Geometry check sheet. Reference: the model listing, model coordinates, mm. Face numbers are marked on the shaded views. A direction names the side the tool comes from. Round coordinates to 2 decimals unless told otherwise and drop trailing zeros. Loops run counter-clockwise (first coordinate to the right, second up) from the corner with the lowest first, then second, coordinate; pieces in that order, holes last.
Autodesk Fusion 360 part; units mm, degrees
sketch "Sketch1" plane through (0, 0, 0) normal (0, 1, 0) x (1, 0, 0)
  line L0 (0, 64.0421) -> (0, -79.964)
  line L1 (-3.05, -8) -> (-3.05, 0)
  line L2 (-6.25, 0) -> (-6.25, 12)
  line L3 (-6.25, 0) -> (-3.05, 0)
  line L4 (-8.05, -8) -> (-8.05, -5)
  line L5 (-11.25, -5) -> (-8.05, -5)
  line L6 (-11.25, -5) -> (-11.25, 12)
  line L7 (-8.05, -8) -> (-3.05, -8)
  line L8 (-11.25, 12) -> (-6.25, 12)
  line L9 (-3.05, -8) -> (0, -7.961)
  line L10 (-6.25, 12) -> (0, 12)
  dimension "d1" = 12.5
  dimension "d2" = 6.1
  dimension "d3" = 8
  dimension "d7" = 12
  dimension "d8" = -5
revolve "Revolve1" add sketch "Sketch1" angle 360 about axis through (0, 0, -64.0421) along (0, 0, 1)
sketch "Sketch2" plane through (0, 0, 8) normal (0, 0, 1) x (-1, 0, 0)
  circle A0 centre (0, 0) radius 3.05 construction
  circle A1 centre (0, 0) radius 8.05
  line L0 (-3.05, 3.05) -> (3.05, 3.05)
  line L1 (3.05, 3.05) -> (3.05, -3.05)
  line L2 (3.05, -3.05) -> (-3.05, -3.05)
  line L3 (-3.05, -3.05) -> (-3.05, 3.05)
  line L4 (-3.05, 3.05) -> (3.05, -3.05) construction
  line L5 (3.05, 3.05) -> (-3.05, -3.05) construction
  point P0 (3.05, 0)
extrude "Extrude1" cut sketch "Sketch2" against normal through all contours L0 L1 L2 L3
sketch "Sketch3" plane through (0, 0, -12) normal (0, 0, -1) x (1, 0, 0)
  line L0 (3.05, 3.05) -> (3.05, -3.05)
  line L1 (3.05, -3.05) -> (-3.05, -3.05)
  line L2 (-3.05, -3.05) -> (-3.05, 3.05)
  line L3 (-3.05, 3.05) -> (3.05, 3.05)
  circle A0 centre (0, 0) radius 11.25
  line L4 (-6, 6) -> (6, 6)
  line L5 (6, 6) -> (6, -6)
  line L6 (6, -6) -> (-6, -6)
  line L7 (-6, -6) -> (-6, 6)
  line L8 (-6, 6) -> (6, -6) construction
  line L9 (6, 6) -> (-6, -6) construction
  dimension "d11" = 12
  dimension "d12" = 12
extrude "Extrude2" cut sketch "Sketch3" against normal blind 12 contours L4 L5 L6 L7
chamfer "Chamfer1" distance 1.9 angle 45 1 edges at (-7.5052, 2.911, 5)
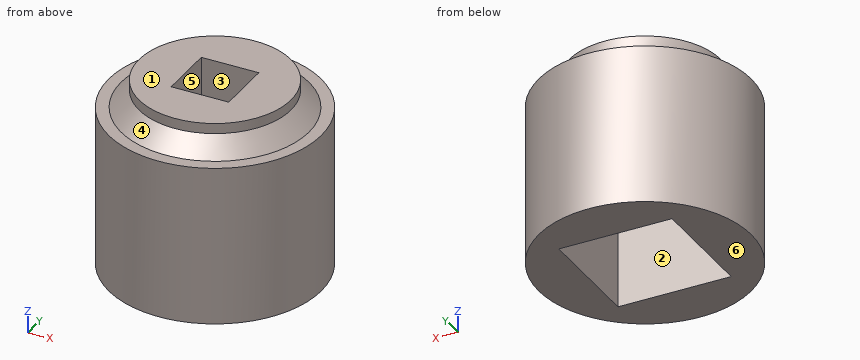
1) Mould release check, pull along X, two halves, no side actions. Record for the marked faces 4, 5 and 6: +X half, -X half, draft (parallel to the pull), parting line (faces both ways), or undercut.
Report:
face 4: parting line
face 5: undercut
face 6: draft
2) Scan lines: line 1 along Z through (x, y) = (4.5, -5); line 2 along X through (y, z) = (4.25, -3.5); line 3 along X through (y, z) = (4.5, -7). Record each from-to range of solid material in increasing order.
Report:
line 1: z = 0 to 8
line 2: x = -10.42 to -6, 6 to 10.42
line 3: x = -10.31 to -6, 6 to 10.31
3) Sectioned sample at A-A, the plane x = 0. Record the cut outline in (y, z), then the cut area to 3 significant figures.
Report:
outline: (-11.25, -12) - (-6, -12) - (-6, 0) - (-3.05, 0) - (-3.05, 8) - (-8.05, 8) - (-8.05, 6.9) - (-9.95, 5) - (-11.25, 5) - close; (3.05, 0) - (6, 0) - (6, -12) - (11.25, -12) - (11.25, 5) - (9.95, 5) - (8.05, 6.9) - (8.05, 8) - (3.05, 8) - close
area: 242 mm2
4) Gauge pin test, flat ends, axial feed: pin 1 (3.5 mm diameter, centred on x = 2, z = -8, fed in from -Y); pin 2 (3.5 mm diameter, centred on y = -2, z = -3, fed in from +X); pin 3 (6 mm diameter, centred on x = -2, y = -1.5, fed in from -Z). Record the tip position at first contact, or that the pin passes through.
Report:
pin 1: stops at y = -11.25
pin 2: stops at x = 11.25
pin 3: stops at z = 0
5) Access from +Z, -Z, +X, -X, +Y, -Y to the whole of each face (thin tool, end or side, straight path). Record for the marked faces 1, 2 and 3.
Report:
face 1: +Z, +X, -X, +Y, -Y
face 2: -Z
face 3: +Z, -Z
6) Sectioned sample at C-C, the plane z = 6.25. Record the cut outline in (x, y).
Report:
outline: circle Ø17.4 at (0, 0); hole (-3.05, -3.05) - (3.05, -3.05) - (3.05, 3.05) - (-3.05, 3.05) - close
7) Sectioned sample at D-D, the plane z = -7. Record the cut outline in (x, y).
Report:
outline: circle Ø22.5 at (0, 0); hole (-6, -6) - (6, -6) - (6, 6) - (-6, 6) - close
